Drawing for the job (mm, zero at the part's lowest x, y, z). Round coordinates to 2 decimals unless told otherwise and drop trailing zeros. Loops run counter-clockwise (first coordinate to the right, second up) from the corner with the lowest first, then second, coordinate; pieces in that order, holes last. Notation, with made-up numbers: (63, 61) -> (97, 61) arc R15 ccw to (97, 88) -> close; hole circle Ø11 at (-13, -16.5). An arc over 180 degrees is marked (long way). Put each result on its own line as item: value. Start each with the question number.
Item 1: Flat gauge pins, fed straight in: pin 1 Ø2.5 at (x, y) = (3.5, 160.5) entering from -Z (1 decimal); pin 2 Ø2.5 at (x, y) = (3.5, 60) entering from -Z; pin 3 Ø2.5 at (x, z) = (2, 189) entering from -Y; pin 4 Ø1.5 at (x, y) = (2.5, 160.5) entering from +Z (1 decimal). Where does each tip first touch, or does it go through?
Item 2: Cut at C-C, the plane x = 3.1. Count the separate pieces of the cut face and the enclosed holes in it, plus the area to 3 significant figures.
Item 3: Cut at A-A, the plane z = 101.6. List the corners of the cut face in (x, y) (1 decimal).
Item 4: Cut at B-B, the plane y = 61. List the corners of the cut face in (x, z) (1 decimal).
Item 5: Cut at D-D, the plane z = 81. List the corners of the cut face in (x, y) (1 decimal).
Item 6: Drill centre lines: probe 1 along Y at (x, z) = (1.5, 29) (1 decimal); probe 2 along Y at (x, z) = (1.45, 86.1) (1 decimal); probe 3 along Y at (x, z) = (1.35, 101.6). Where is each one in solid material? Low to high. Write a range as [from, to].
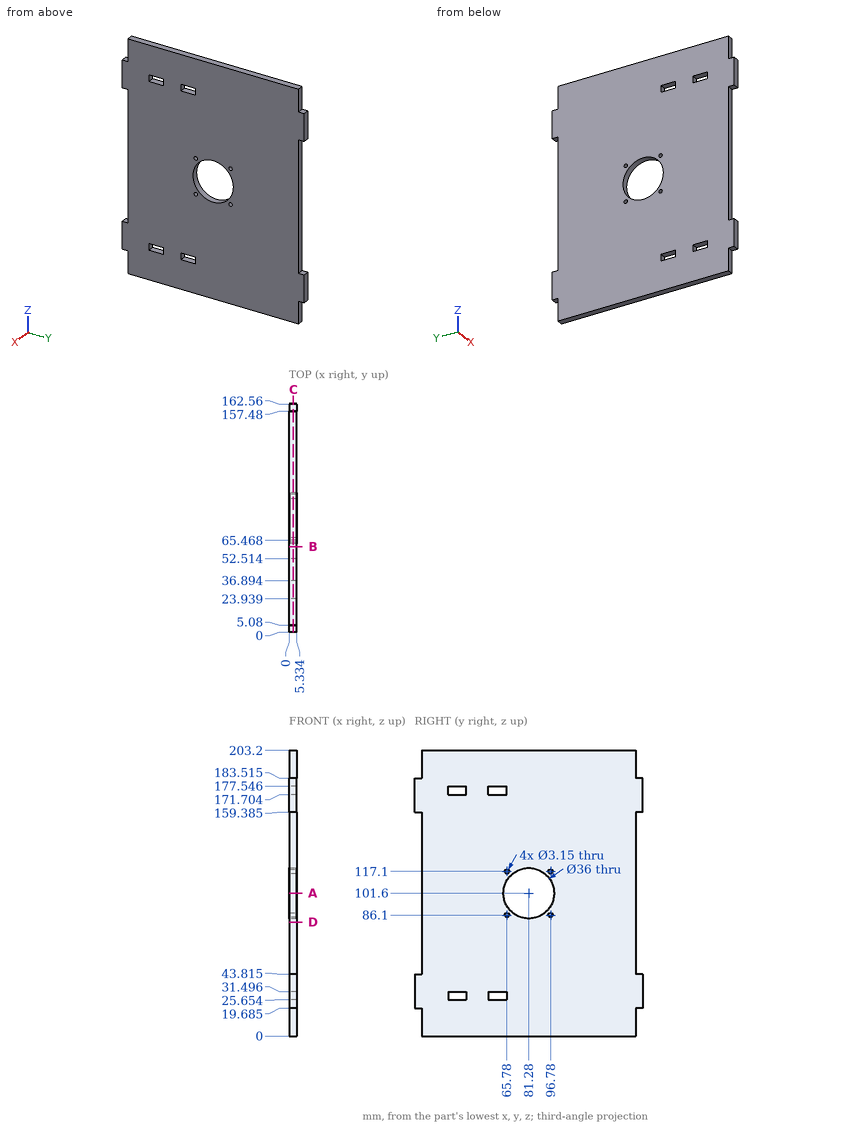
Reply:
1. pin 1: stops at z = 19.7
1. pin 2: stops at z = 0
1. pin 3: stops at y = 5.08
1. pin 4: stops at z = 183.5
2. separate pieces: 1
2. enclosed holes: 9
2. area: 30,100 mm^2
3. outline: (0, 5.1) -> (5.3, 5.1) -> (5.3, 63.3) -> (0, 63.3) -> close; (0, 99.3) -> (5.3, 99.3) -> (5.3, 157.5) -> (0, 157.5) -> close
4. outline: (0, 0) -> (5.3, 0) -> (5.3, 25.7) -> (0, 25.7) -> close; (0, 31.5) -> (5.3, 31.5) -> (5.3, 171.7) -> (0, 171.7) -> close; (0, 177.5) -> (5.3, 177.5) -> (5.3, 203.2) -> (0, 203.2) -> close
5. outline: (0, 5.1) -> (5.3, 5.1) -> (5.3, 157.5) -> (0, 157.5) -> close
6. probe 1: y = [0, 23.9], [36.9, 52.5], [65.5, 162.6]
6. probe 2: y = [5.1, 64.2], [67.4, 72.1], [90.4, 95.2], [98.4, 157.5]
6. probe 3: y = [5.08, 63.28], [99.28, 157.48]
